Geometry: final body of the model. Coordinates: model frame, mm. Face numbers are marked on the shaded views. Give positions to 0.01 mm unless a question says otherwise; leave off trailing zeros. Loops run counter-clockwise (first coordinate to the right, second up) from the corner with the lowest first, then second, coordinate; pieces in that order, holes last. Notation, with made-up numbers: (58, 50) - (93, 50) arc R32 cw to (93, 78) - close; hole circle Ø10 at (10, 45). An arc over 180 degrees is marked (long way). Answer in a Markdown table with one row per item.
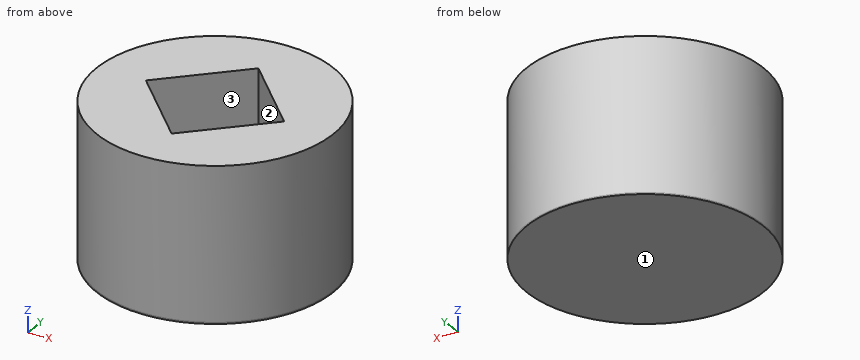
from build123d import *

# Parameters (mm, degrees)
F0_R     = 39.37
F1_DEPTH = 0.508
F2_R     = 39.37
F3_DEPTH = 50.8
F5_DEPTH = 33.02


with BuildPart() as f1:
    # F0 (on Top) → F1 (new body)
    with BuildSketch(Plane.XY):
        Circle(F0_R)
    extrude(amount=-F1_DEPTH)

    # F2 (on Top) → F3 (join)
    with BuildSketch(Plane.XY):
        Circle(F2_R)
    extrude(amount=F3_DEPTH)

    # F4 (on face) → F5 (cut)
    with BuildSketch(Plane.XY.offset(50.8)):
        Polygon((23.348666, 0), (0, 23.348666), (-23.348666, 0), (0, -23.348666), align=None)
    extrude(amount=-F5_DEPTH, mode=Mode.SUBTRACT)


solid = f1.part
Q1. Cut plane D-D (y = 24.5). Output: boundary loops of the cut face in (x, z), and give its area (3 significant figures).
Check values:
| item | result |
|---|---|
| outline | (-30.82, -0.51) - (30.82, -0.51) - (30.82, 50.8) - (-30.82, 50.8) - close |
| area | 3,160 mm² |
Q2. First-contact query: pin 1 (1.5 mm diameter, centred on y = -20, z = 23.5, fed in from -X); pin 2 (3 mm diameter, centred on x = -24, z = 38, fed in from +Y); pin 3 (10 mm diameter, centred on x = -15.5, z = 24, fed in from +Y). Flat tips, straight axial feed; report the tip coordinate or a pass-through.
Check values:
| item | result |
|---|---|
| pin 1 | x = -34.34 |
| pin 2 | y = 32.31 |
| pin 3 | y = 37.94 |
Q3. Cut plane A-A (z = 24). Output: boundary loops of the cut face in (x, y), and give its area (3 significant figures).
Check values:
| item | result |
|---|---|
| outline | circle Ø78.74 at (0, 0); hole (-23.35, 0) - (0, -23.35) - (23.35, 0) - (0, 23.35) - close |
| area | 3,780 mm² |
Q4. Cut plane C-C (y = -1). Output: boundary loops of the cut face in (x, z).
Check values:
| item | result |
|---|---|
| outline | (-39.36, -0.51) - (39.36, -0.51) - (39.36, 50.8) - (22.35, 50.8) - (22.35, 17.78) - (-22.35, 17.78) - (-22.35, 50.8) - (-39.36, 50.8) - close |
Q5. Draft query along X for the marked faces 1, 2 and 3. Return one class per face: pulls with the +X half, pulls with the -X half, needs draft (parallel to the pull), parting line crosses it, or undercut.
Check values:
| item | result |
|---|---|
| face 1 | needs draft |
| face 2 | undercut |
| face 3 | undercut |
Q6. Cut plane B-B (x = -9). Output: boundary loops of the cut face in (y, z).
Check values:
| item | result |
|---|---|
| outline | (-38.33, -0.51) - (38.33, -0.51) - (38.33, 50.8) - (14.35, 50.8) - (14.35, 17.78) - (-14.35, 17.78) - (-14.35, 50.8) - (-38.33, 50.8) - close |
Q7. Material intervals for line 1 along Z through (x, y) = (-17.5, -0.5); line 2 along Y through (x, z) = (-2, 32); line 3 along X through (y, z) = (-1, 46.5), sorted ascending.
Check values:
| item | result |
|---|---|
| line 1 | -0.51 to 17.78 |
| line 2 | -39.32 to -21.35, 21.35 to 39.32 |
| line 3 | -39.36 to -22.35, 22.35 to 39.36 |
